```python
from build123d import *

# Parameters (mm, degrees)
ESQUISSE1_R        = 1.5
BOSS_EXTRU_1_DEPTH = 5
CONG_1_R           = 6


with BuildPart() as part:
    # Esquisse1 → Boss.-Extru.1 (new body)
    with BuildSketch(Plane.XY):
        with BuildLine():
            Line((0, 8), (5, 8))
            Line((5, 8), (20, 5))
            Line((20, 5), (20, -8))
            Line((20, -8), (0, -8))
            ThreePointArc((0, -8), (-8, 0), (0, 8))
        make_face()
        Circle(ESQUISSE1_R, mode=Mode.SUBTRACT)
        with Locations((15, 0)):
            Circle(ESQUISSE1_R, mode=Mode.SUBTRACT)
    extrude(amount=BOSS_EXTRU_1_DEPTH)

    # Congé1
    cong_1_edges = [part.edges().sort_by_distance(p)[0] for p in [
        (20, 5, 2.5),
    ]]
    fillet(cong_1_edges, radius=CONG_1_R)


solid = part.part
```
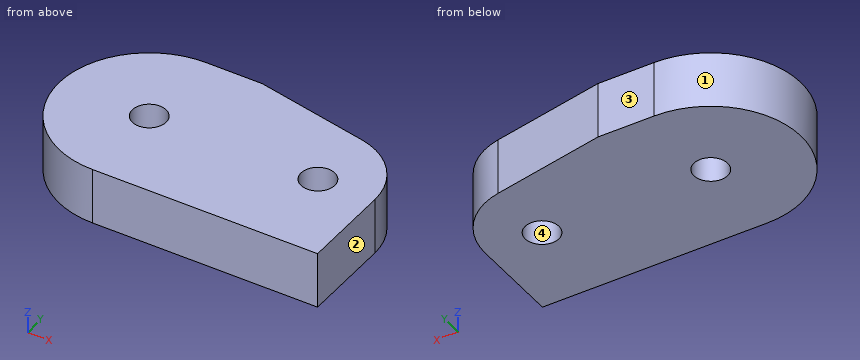
Geometry: final body of the model. Coordinates: model frame, mm. Face numbers are marked on the shaded views. Coordinates: 2 decimals unless noted, no trailing zeros. Write each loop counter-clockwise with the first axis right and the second up, starting at its lowest first coordinate (ties: lowest second). Pieces come first, ordered by that corner, then holes. Notation, with made-up numbers: M -16,32 L 32,32 A23 cw 32,68 Z; hole C 54,16.5 d9. An arc over 180 degrees is marked long. Use CSV: the item, a comma, the result in double quotes. Start each with the question number.
1. Mould query, pull axis X, two halves, no side actions, for the marked faces 1, 2, 3 and 4. Classes: pulls with the +X half, pulls with the -X half, needs draft (parallel to the pull), parting line crosses it, or undercut.
2. Cut plane C-C on y = -3.75. Return the cut outline in (x, z).
3. Cut plane B-B on x = 9.5. Return the cut outline in (y, z).
4. Cut plane A-A on z = 4.5. Return the cut outline in (x, y).
5. Ray query, probe 1 along Y at (x, z) = (0, 2.95); probe 2 along X at (y, z) = (1, 1.5); probe 3 along X at (y, z) = (1.25, 0.7). Return the intervals inside material, ascending.
6. First-contact query: P1, Ø5, axis at x = 15, y = 0, coming from the +Z side; P2, Ø1.5, axis at y = 1, z = 4.5, coming from the -X side; P3, Ø3, axis at y = 5, z = 3, coming from the +X side; P4, Ø1, axis at y = 4, z = 4, coming from the -X side. Flat tips, straight axial feed; report the tip coordinate or a pass-through.
Entries:
1,face 1,"pulls with the -X half"
1,face 2,"pulls with the +X half"
1,face 3,"needs draft"
1,face 4,"undercut"
2,outline,"M -7.07,0 L 20,0 L 20,5 L -7.07,5 Z"
3,outline,"M -8,0 L 7.1,0 L 7.1,5 L -8,5 Z"
4,outline,"M 0,-8 L 20,-8 L 20,0.08 A6 ccw 15.18,5.96 L 5,8 L 0,8 A8 ccw Z; hole C 0,0 d3; hole C 15,0 d3"
5,probe 1,"-8 to -1.5, 1.5 to 8"
5,probe 2,"-7.94 to -1.12, 1.12 to 13.88, 16.12 to 19.93"
5,probe 3,"-7.9 to -0.83, 0.83 to 14.17, 15.83 to 19.89"
6,P1,"z = 5"
6,P2,"x = -8"
6,P3,"x = 18.93"
6,P4,"x = -7.19"
